Autodesk Inventor part; units mm, degrees
ref_plane "YZ Plane" through (0, 0, 0) normal (1, 0, 0) x (0, 1, 0)
ref_plane "XZ Plane" through (0, 0, 0) normal (0, 1, 0) x (-1, 0, 0)
ref_plane "XY Plane" through (0, 0, 0) normal (0, 0, 1) x (1, 0, 0)
sketch "Sketch1" plane through (0, 0, 0) normal (0, 1, 0) x (-1, 0, 0)
  line L0 (18, 38.5) -> (-18, 38.5)
  line L1 (-18, 38.5) -> (-18, -38.5)
  line L2 (-18, -38.5) -> (18, -38.5)
  line L3 (18, -38.5) -> (18, 38.5)
  line L4 (18, 38.5) -> (-18, -38.5) construction
  point P0 (0, 0)
  point P1 (0, 0)
  dimension "d0" = 77
  dimension "d1" = 36
extrude "Extrusion1" add sketch "Sketch1" along normal blind 122
sketch "Sketch2" plane through (0, 122, 0) normal (0, 1, 0) x (1, 0, 0)
  line L0 (-30.5, -50) -> (30.5, -50)
  line L1 (30.5, -50) -> (30.5, 50)
  line L2 (30.5, 50) -> (-30.5, 50)
  line L3 (-30.5, 50) -> (-30.5, -50)
  line L4 (-30.5, 50) -> (30.5, -50) construction
  point P0 (0, 0)
  point P1 (0, 0)
  dimension "d4" = 100
  dimension "d5" = 61
extrude "Extrusion2" add sketch "Sketch2" along normal blind 19
sketch "Sketch3" plane through (0, 141, 0) normal (0, 1, 0) x (1, 0, 0)
  circle A0 centre (0, 0) radius 17
  dimension "d8" = 34
extrude "Extrusion3" add sketch "Sketch3" along normal blind 53
sketch "Sketch4" plane through (0, 194, 0) normal (0, 1, 0) x (1, 0, 0)
  line L0 (-30, -30) -> (30, -30)
  line L1 (30, -30) -> (30, 30)
  line L2 (30, 30) -> (-30, 30)
  line L3 (-30, 30) -> (-30, -30)
  line L4 (-30, 30) -> (30, -30) construction
  point P0 (0, 0)
  point P1 (0, 0)
  dimension "d11" = 60
extrude "Extrusion4" add sketch "Sketch4" along normal blind 126
sketch "Sketch5" plane through (-30, 194, 30) normal (0, 0, 1) x (1, 0, 0)
  circle A0 centre (30, 14) radius 7.5
  line L0 (0, 0) -> (60, 0)
  circle A1 centre (30, 121) radius 7.5
  line L1 (0, 126) -> (60, 126)
  point P0 (30, -194)
  point P1 (30, 0)
  point P2 (30, 126)
  point P3 (35.5902, 126)
  point P4 (24.4098, 126)
  dimension "d14" = 15
  dimension "d15" = 14
  dimension "d16" = 5
extrude "Extrusion5" add sketch "Sketch5" along normal blind 40
chamfer "Chamfer1" distance 5 angle 45 4 edges at (30, 257, 30) (30, 257, -30) (-30, 257, -30) (-30, 257, 30)
chamfer "Chamfer2" distance 5 angle 45 4 edges at (30.5, 131.5, -50) (-30.5, 131.5, -50) (-30.5, 131.5, 50) (30.5, 131.5, 50)
fillet "Fillet1" radius 8 2 edges at (0, 0, 38.5) (0, 0, -38.5)
sketch "Sketch6" plane through (18, 122, 38.5) normal (1, 0, 0) x (0, 0, -1)
  circle A0 centre (38.5, -83) radius 34.5
  line L0 (8, -122) -> (69, -122)
  point P0 (38.5, -122)
  point P1 (38.5, -122)
  dimension "d26" = 39
  dimension "d27" = 69
extrude "Extrusion6" cut sketch "Sketch6" against normal through all
properties part number "Gatevalve_70_pneumatic" material "Stainless Steel, 440C"
The listing builds one solid part. Answer for the finished solid, in the listing's coordinates (mm). A direction names the side the tool comes from. Round coordinates to 2 decimals unless told otherwise and drop trailing zeros. Order: outer loops, then holes, each group sorted by start corner. A loop starts at its lowest first (then second) coordinate and runs counter-clockwise, first axis right, second up. Notation, with made-up numbers: (5, 45.5) - (64, 45.5) arc R29 cw to (64, 69.5) - close; hole circle Ø4 at (36.5, 26). An arc over 180 degrees is marked (long way). Write item = value, one per line. Start each with the question number.
1) Straight lines are drawn through the part: L1, parallel to Y at x = 21.5, z = 4.5; L2, parallel to Y at x = 3, z = 0.5; L3, parallel to Z at x = -13.5, y = 220. For each, find the intervals that lie inside material, in ascending order.
2) Section A-A, the plane y = 39 is taken. Write down the section's boundary in (x, z).
3) For faces 4 (the cylindrical face through (-1.63, 322.32, 49.72)), 5 (the flat face through (0, 64, 38.5)), 6 (the flat face through (-14, 194, -14)), 7 (the flat face through (0, 256, -30)), 8 (the flat face through (-30, 256, 0)), determine the directions among +Z, -Z, +X, -X, +Y, -Y from which every point of the face is accessible in a straight line to the end or side of a thin tool.
4) Section C-C, the plane z = 0 is taken. Write down the section's boundary in (x, y).
5) Section B-B, the plane x = 0 is taken. Write down the section's boundary in (y, z), plus the area to 3 significant figures.
6) Given pin 1 (23 mm diameter, centred on y = 73.5, z = 8, fed in from +X); pin 2 (8 mm diameter, centred on x = 23, z = 28.5, fed in from +Y); pin 3 (15 mm diameter, centred on x = 7.5, y = 288, fed in from -Z), each flat-ended and moving along its own axis, determine where each tip first touches the part or whether it passes through.
7) Section D-D, the plane y = 315 is taken. Write down the section's boundary in (x, z), plus the area to 3 significant figures.
8) For a pull along Y with two mould halves and no side action, classify faces 1 (the cylindrical face through (0.25, 68.09, -18.55)), 2 (the flat face through (18, 74, 1)), 3 (the cylindrical face through (-0.252, 2.406, -36.219)) as released by +Y, released by -Y, zero draft, split by the parting line, or undercut.
Results list:
q1.L1 = 122 to 141, 194 to 320
q1.L2 = 0 to 4.5, 73.5 to 320
q1.L3 = -30 to 30
q2.outline = (-18, -38.5) - (18, -38.5) - (18, -34.5) - (-18, -34.5) - close; (-18, 34.5) - (18, 34.5) - (18, 38.5) - (-18, 38.5) - close
q3.face_4 = +Z
q3.face_5 = +Z, +X, -X, -Y
q3.face_6 = none
q3.face_7 = -Z, +X, -X, +Y
q3.face_8 = +Z, -Z, -X, +Y
q4.outline = (-30.5, 122) - (-18, 122) - (-18, 73.5) - (18, 73.5) - (18, 122) - (30.5, 122) - (30.5, 141) - (17, 141) - (17, 194) - (30, 194) - (30, 320) - (-30, 320) - (-30, 194) - (-17, 194) - (-17, 141) - (-30.5, 141) - close; (-18, 0) - (18, 0) - (18, 4.5) - (-18, 4.5) - close
q5.outline = (0, -30.5) arc R8 ccw to (8, -38.5) - (122, -38.5) - (122, -50) - (141, -50) - (141, -17) - (194, -17) - (194, -30) - (320, -30) - (320, 30) - (322.5, 30) - (322.5, 70) - (307.5, 70) - (307.5, 30) - (215.5, 30) - (215.5, 70) - (200.5, 70) - (200.5, 30) - (194, 30) - (194, 17) - (141, 17) - (141, 50) - (122, 50) - (122, 38.5) - (8, 38.5) arc R8 ccw to (0, 30.5) - close; hole circle Ø69 at (39, 0)
q5.area = 18,100 mm^2
q6.pin_1 = 18
q6.pin_2 = 320
q6.pin_3 = -30
q7.outline = (-30, -25) - (-25, -30) - (25, -30) - (30, -25) - (30, 25) - (25, 30) - (7.5, 30) - (7.5, 70) - (-7.5, 70) - (-7.5, 30) - (-25, 30) - (-30, 25) - close
q7.area = 4,150 mm^2
q8.face_1 = undercut
q8.face_2 = zero draft
q8.face_3 = released by -Y
